from build123d import *

# Parameters (mm, degrees)
F0_W     = 6.35
F0_H     = 9.525
F1_DEPTH = 3.175


with BuildPart() as f1:
    # F0 (on Top) → F1 (new body)
    with BuildSketch(Plane.XY):
        Polygon((6.35, 9.525), (6.35, 0), (63.5, 50.8), (0, 13.277273), align=None)
        Polygon((-63.5, 50.8), (-6.35, 0), (-6.35, 9.525), (0, 13.277273), align=None)
        Polygon((0, 13.277273), (-6.35, 9.525), (0, 9.525), align=None)
        Polygon((0, 9.525), (6.35, 9.525), (0, 13.277273), align=None)
        with Locations((-3.175, 4.7625)):
            Rectangle(F0_W, F0_H)
        with Locations((3.175, 4.7625)):
            Rectangle(F0_W, F0_H)
        Polygon((-6.35, -9.525), (6.35, -9.525), (6.35, 0), (0, 0), (-6.35, 0), align=None)
    extrude(amount=F1_DEPTH)


solid = f1.part
For this review, take the finished solid that the model builds, in its own axes (mm). A direction names the side the tool comes from. Coordinates: 2 decimals unless noted, no trailing zeros. Order: outer loops, then holes, each group sorted by start corner. A loop starts at its lowest first (then second) coordinate and runs counter-clockwise, first axis right, second up. Notation, with made-up numbers: (62, 33.5) -> (82, 33.5) arc R32 cw to (82, 67.5) -> close; hole circle Ø1 at (29.25, 61.25). An arc over 180 degrees is marked (long way). Return JSON: item names as keys, results as strings.
1. Machinability: for faces 1 (the flat face through (6.35, -5, 2)), 2 (the flat face through (0, -9.525, 2)), which of the approach directions +Z, -Z, +X, -X, +Y, -Y give a long, thin tool a straight path to every point of the face, cutting with its end or side? Answer none if there is none.
Answer block:
{"face 1": "+Z, -Z, +X, -Y", "face 2": "+Z, -Z, +X, -X, -Y"}
2. For pin 1 Ø1.5 at (y, z) = (-3, 2) entering from -X; pin 2 Ø1 at (x, z) = (46.5, 0.5) entering from +Y; pin 3 Ø1.5 at (x, z) = (-40, 2) entering from +Y, all flat-tipped, find the tip position at first contact; note any pin that passes through.
Answer block:
{"pin 1": "x = -6.35", "pin 2": "y = 41.05", "pin 3": "y = 37.36"}
3. We need section A-A on y = 38. Write out the cut boundary in (x, z) (3 decimals), and give its area (3 significant figures).
Answer block:
{"outline": "(-49.1, 0) -> (-41.838, 0) -> (-41.838, 3.175) -> (-49.1, 3.175) -> close; (41.838, 0) -> (49.1, 0) -> (49.1, 3.175) -> (41.838, 3.175) -> close", "area": "46.1 mm²"}
4. The part is to be moulded in two halves that separate along X. For faces 3 (the flat face through (-6.35, -5, 2)), 4 (the flat face through (-31.31, 31.78, 1.57)), 5 (the flat face through (32.19, 32.3, 1.57)), 6 (the flat face through (4, 14, 0)), say which applies: +X half, -X half, draft (parallel to the pull), parting line (faces both ways), or undercut.
Answer block:
{"face 3": "-X half", "face 4": "undercut", "face 5": "undercut", "face 6": "draft"}
5. We need section B-B on z = 1.35. Write out the cut boundary in (x, y) (3 decimals).
Answer block:
{"outline": "(-63.5, 50.8) -> (-6.35, 0) -> (-6.35, -9.525) -> (6.35, -9.525) -> (6.35, 0) -> (63.5, 50.8) -> (0, 13.277) -> close"}
6. For line 1 (X direction, y = -1.5, z = 2.05); line 2 (X direction, y = 36, z = 2.3), list the stretches that pass through material, from the lowest coordinate up. Write a range as from..to.
Answer block:
{"line 1": "-6.35..6.35", "line 2": "-46.85..-38.45, 38.45..46.85"}
7. We need section C-C on x = 3. Write out the cut boundary in (y, z) (3 decimals).
Answer block:
{"outline": "(-9.525, 0) -> (15.05, 0) -> (15.05, 3.175) -> (-9.525, 3.175) -> close"}
8. We need section D-D on y = 8. Write out the cut boundary in (x, z) (3 decimals), and give its area (3 significant figures).
Answer block:
{"outline": "(-15.35, 0) -> (15.35, 0) -> (15.35, 3.175) -> (-15.35, 3.175) -> close", "area": "97.5 mm²"}
